Read the model definition and answer for the solid it produces. Units are mm, in the model's axes. Face numbers are marked on the shaded views. Coordinates: 2 decimals unless noted, no trailing zeros. Loops run counter-clockwise (first coordinate to the right, second up) from the corner with the lowest first, then second, coordinate; pieces in that order, holes last. Notation, with made-up numbers: M 58,71.25 L 105,71.25 A24 cw 105,104.25 Z; hole C -29.5,-1.75 d2. An arc over 180 degrees is marked long. One line per item, written item: value. Start each with the question number.
1. Flat-ended cylindrical pins translate along their axes: pin 1 (2.5 mm diameter, centred on x = 30, z = -28, fed in from -Y); pin 2 (7 mm diameter, centred on x = 17.25, z = -79.84, fed in from -Y). Find the tip coordinate at first contact, or state that the pin passes through.
2. The part is cut by section D-D (z = -43.5). Write down the section's boundary in (x, y).
3. Consider probe 1 along X at (y, z) = (3.5, -10); probe 2 along X at (y, z) = (0.75, -103.5); probe 3 along X at (y, z) = (4, -66). Determine where each line is inside the solid, lowest interval first.
4. Determine the mould class of the marked faces 1 and 2 for opening direction Z: +Z half, -Z half, draft (parallel to the pull), parting line (faces both ways), or undercut.
5. The part is cut by section B-B (y = 6). State how many separate pieces and enclosed holes the cut face has, then the cut area to 3 significant figures.
6. The part is cut by section C-C (z = -68.5). Write down the section's boundary in (x, y).
7. The part is cut by section A-A (z = -10). Write down the section's boundary in (x, y).
```python
from build123d import *

# Parameters (mm, degrees)
SKETCH1_W                            = 125
SKETCH1_H                            = 115
TOP_BASE_DEPTH                       = 9
SKETCH5_R                            = 14.5
DRIVE_GEAR_EXTRUDE_CUT_DEPTH         = 6
SKETCH17_R                           = 20
INTERMEDIATE_GEAR_TOP_PART_CUT_DEPTH = 171.091152033
SKETCH8_R                            = 17.75
THUMB_EXTRUDE_CUT_DEPTH              = 171.091152033
SKETCH26_R                           = 1.5
STRING_HOLES_DEPTH                   = 171.091152033
THUMB_MOUNT_HOLES_R                  = 2
THUMB_MOUNT_HOLES_M4_DEPTH           = 171.091152033
FINGERS_MOUNT_HOLES_R                = 2
FINGERS_MOUNT_HOLES_M4_DEPTH         = 171.091152033
CONNECT_HOLES_POSITION_R             = 2.8
CONNECT_HOLES_M6_DEPTH               = 171.091152033
SKETCH27_R                           = 3.75
XL320_NUT_M4_DEPTH                   = 4


with BuildPart() as part:
    # Sketch1 → Top_Base (new body)
    with BuildSketch(Plane(origin=(0, 0, 0), x_dir=(1, 0, 0), z_dir=(0, 1, 0))):
        with Locations((62.5, 57.5)):
            Rectangle(SKETCH1_W, SKETCH1_H)
    extrude(amount=TOP_BASE_DEPTH)

    # Sketch5 → Drive_Gear_Extrude_Cut (cut)
    with BuildSketch(Plane(origin=(0, 9, 0), x_dir=(1, 0, 0), z_dir=(0, 1, 0))):
        with Locations(Location((23.25, 55.841914565, 0), (0, 0, 270))):
            Circle(SKETCH5_R)
    extrude(amount=-DRIVE_GEAR_EXTRUDE_CUT_DEPTH, mode=Mode.SUBTRACT)

    # Sketch17 → Intermediate_Gear_Top_Part_Cut (cut, through all)
    with BuildSketch(Plane(origin=(0, 9, 0), x_dir=(1, 0, 0), z_dir=(0, 1, 0))):
        with Locations(Location((53.923140352, 53.049342105, 0), (0, 0, 270))):
            Circle(SKETCH17_R)
    extrude(amount=-INTERMEDIATE_GEAR_TOP_PART_CUT_DEPTH, mode=Mode.SUBTRACT)

    # Sketch8 → Thumb_Extrude_Cut (cut, through all)
    with BuildSketch(Plane(origin=(0, 9, 0), x_dir=(1, 0, 0), z_dir=(0, 1, 0))):
        with Locations(Location((104.5, 57.5, 0), (0, 0, 270))):
            Circle(SKETCH8_R)
    extrude(amount=-THUMB_EXTRUDE_CUT_DEPTH, mode=Mode.SUBTRACT)

    # Sketch26 → String_Holes (cut, through all)
    with BuildSketch(Plane.XZ):
        with Locations(Location((30, -28, 0), (0, 0, 270))):
            Circle(SKETCH26_R)
        with Locations(Location((30, -87, 0), (0, 0, 90))):
            Circle(SKETCH26_R)
    extrude(amount=-STRING_HOLES_DEPTH, mode=Mode.SUBTRACT)

    # Thumb_Mount_Holes → Thumb_Mount_Holes_(M4) (cut, through all)
    with BuildSketch(Plane(origin=(0, 9, 0), x_dir=(1, 0, 0), z_dir=(0, 1, 0))):
        with Locations(Location((104.5, 110, 0), (0, 0, 270))):
            Circle(THUMB_MOUNT_HOLES_R)
        with Locations(Location((85, 103, 0), (0, 0, 270))):
            Circle(THUMB_MOUNT_HOLES_R)
        with Locations(Location((110.5, 33.5, 0), (0, 0, 270))):
            Circle(THUMB_MOUNT_HOLES_R)
        with Locations(Location((98.5, 33.5, 0), (0, 0, 90))):
            Circle(THUMB_MOUNT_HOLES_R)
    extrude(amount=-THUMB_MOUNT_HOLES_M4_DEPTH, mode=Mode.SUBTRACT)

    # Fingers_Mount_Holes → Fingers_Mount_Holes_(M4) (cut, through all)
    with BuildSketch(Plane(origin=(0, 9, 0), x_dir=(1, 0, 0), z_dir=(0, 1, 0))):
        with Locations(Location((67.75, 96, 0), (0, 0, 270))):
            Circle(FINGERS_MOUNT_HOLES_R)
        with Locations(Location((67.75, 19, 0), (0, 0, 90))):
            Circle(FINGERS_MOUNT_HOLES_R)
        with Locations(Location((17.25, 79.841914565, 0), (0, 0, 270))):
            Circle(FINGERS_MOUNT_HOLES_R)
        with Locations(Location((29.25, 79.841914565, 0), (0, 0, 90))):
            Circle(FINGERS_MOUNT_HOLES_R)
    extrude(amount=-FINGERS_MOUNT_HOLES_M4_DEPTH, mode=Mode.SUBTRACT)

    # Connect_Holes_Position → Connect_Holes_(M6) (cut, through all)
    with BuildSketch(Plane(origin=(0, 9, 0), x_dir=(1, 0, 0), z_dir=(0, 1, 0))):
        with Locations(Location((10, 105, 0), (0, 0, 270))):
            Circle(CONNECT_HOLES_POSITION_R)
        with Locations(Location((115, 10, 0), (0, 0, 270))):
            Circle(CONNECT_HOLES_POSITION_R)
        with Locations(Location((10, 10, 0), (0, 0, 270))):
            Circle(CONNECT_HOLES_POSITION_R)
    extrude(amount=-CONNECT_HOLES_M6_DEPTH, mode=Mode.SUBTRACT)

    # Sketch27 → XL320_Nut_(M4) (cut)
    with BuildSketch(Plane.XZ):
        with Locations(Location((29.25, -79.841914565, 0), (0, 0, 270))):
            Circle(SKETCH27_R)
        with Locations(Location((17.25, -79.841914565, 0), (0, 0, 270))):
            Circle(SKETCH27_R)
    extrude(amount=-XL320_NUT_M4_DEPTH, mode=Mode.SUBTRACT)


solid = part.part
```
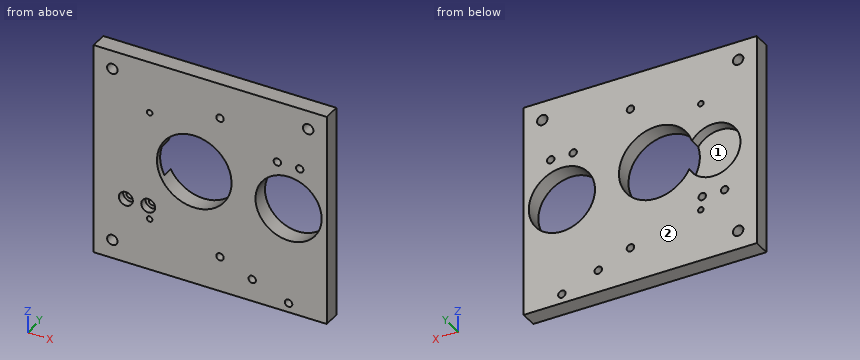
Answer block:
1. pin 1: passes through
1. pin 2: stops at y = 4
2. outline: M 0,0 L 36.35,0 L 36.35,9 L 30.86,9 L 30.86,3 L 15.64,3 L 15.64,9 L 0,9 Z; M 71.5,0 L 93.59,0 L 93.59,9 L 71.5,9 Z; M 115.41,0 L 125,0 L 125,9 L 115.41,9 Z
3. probe 1: x = 0 to 7.2, 12.8 to 112.2, 117.8 to 125
3. probe 2: x = 0 to 7.64, 12.36 to 83.06, 86.94 to 125
3. probe 3: x = 0 to 12.9, 33.6 to 38.68, 69.16 to 88.92, 120.08 to 125
4. face 1: undercut
4. face 2: draft
5. separate pieces: 1
5. enclosed holes: 15
5. area: 11,300 mm2
6. outline: M 0,0 L 41.22,0 L 41.22,9 L 30.32,9 L 30.32,3 L 16.18,3 L 16.18,9 L 0,9 Z; M 66.62,0 L 90.57,0 L 90.57,9 L 66.62,9 Z; M 118.43,0 L 125,0 L 125,9 L 118.43,9 Z
7. outline: M 0,0 L 7.2,0 L 7.2,9 L 0,9 Z; M 12.8,0 L 112.2,0 L 112.2,9 L 12.8,9 Z; M 117.8,0 L 125,0 L 125,9 L 117.8,9 Z
